```python
from build123d import *

# Parameters (mm, degrees)
SKETCH2_R                     = 30
BOSS_EXTRUDE1_DEPTH           = 20
CUT_EXTRUDE2_DEPTH            = 47.904157598
CUT_EXTRUDE3_START            = -10
CUT_EXTRUDE3_DEPTH            = 10
CBORE_FOR_M3_SHCS1_AT_2_COUNT = 2
CBORE_FOR_M3_SHCS1_AT_2_PITCH = 33.587572106
CBORE_FOR_M3_SHCS1_AT_3_COUNT = 2
CBORE_FOR_M3_SHCS1_AT_3_PITCH = 47.5
SKETCH6_R                     = 2.085
BOSS_EXTRUDE2_DEPTH           = 3


with BuildPart() as part:
    # Sketch2 → Boss-Extrude1 (new body)
    with BuildSketch(Plane(origin=(0, 0, 0), x_dir=(1, 0, 0), z_dir=(0, 1, 0))):
        with Locations(Location((0, 0, 0), (0, 0, 270))):
            Circle(SKETCH2_R)
    extrude(amount=BOSS_EXTRUDE1_DEPTH)

    # Sketch3 → Cut-Extrude2 (cut, through all)
    with BuildSketch(Plane(origin=(0, 20, 0), x_dir=(1, 0, 0), z_dir=(0, 1, 0))):
        with BuildLine():
            ThreePointArc((0, -17.5), (17.5, 0), (0, 17.5))
            Line((0, 17.5), (-2, 17.5))
            Line((-2, 17.5), (-2, 9.2))
            Line((-2, 9.2), (-2, 5.4))
            Line((-2, 5.4), (-8, 0))
            Line((-8, 0), (-2, -5.4))
            Line((-2, -5.4), (-2, -9.2))
            Line((-2, -9.2), (-2, -17.5))
            Line((-2, -17.5), (0, -17.5))
        make_face()
    extrude(amount=-CUT_EXTRUDE2_DEPTH, mode=Mode.SUBTRACT)

    # Sketch3_3 → Cut-Extrude3 (cut)
    with BuildSketch(Plane(origin=(0, 20, 0), x_dir=(1, 0, 0), z_dir=(0, 1, 0)).offset(CUT_EXTRUDE3_START)):
        with BuildLine():
            Line((-17.6, 17.5), (-24.366985862, 17.5))
            ThreePointArc((-24.366985862, 17.5), (-30, 0), (-24.366985862, -17.5))
            Line((-24.366985862, -17.5), (-17.6, -17.5))
            Line((-17.6, -17.5), (-17.6, -21.5))
            Line((-17.6, -21.5), (0, -21.5))
            Line((0, -21.5), (0, -17.5))
            Line((0, -17.5), (-2, -17.5))
            Line((-2, -17.5), (-2, -9.2))
            ThreePointArc((-2, -9.2), (-6.53919762, -12.379149415), (-11.966443699, -13.5))
            Line((-11.966443699, -13.5), (-22, -13.5))
            Line((-22, -13.5), (-22, -9.5))
            Line((-22, -9.5), (-10, -9.5))
            Line((-10, -9.5), (-10, -2))
            Line((-10, -2), (-22, -2))
            Line((-22, -2), (-22, 2))
            Line((-22, 2), (-10, 2))
            Line((-10, 2), (-10, 9.5))
            Line((-10, 9.5), (-22, 9.5))
            Line((-22, 9.5), (-22, 13.5))
            Line((-22, 13.5), (-11.966443699, 13.5))
            ThreePointArc((-11.966443699, 13.5), (-6.53919762, 12.379149415), (-2, 9.2))
            Line((-2, 9.2), (-2, 17.5))
            Line((-2, 17.5), (0, 17.5))
            Line((0, 17.5), (0, 21.5))
            Line((0, 21.5), (-17.6, 21.5))
            Line((-17.6, 21.5), (-17.6, 17.5))
        make_face()
    extrude(amount=CUT_EXTRUDE3_DEPTH, mode=Mode.SUBTRACT)

    # Sketch5 → CBORE for M3 SHCS1 (revolve, cut)
    with BuildSketch(Plane(origin=(0, 0, -23.75), x_dir=(0, 0, -1), z_dir=(1, 0, 0))):
        Polygon((0, 0), (0, 20), (1.7, 20), (1.7, 3), (3.25, 3), (3.25, 0.025), (3.275, 0), align=None)
    cbore_for_m3_shcs1 = revolve(axis=Axis((0, -6.35, -23.75), (0, 1, 0)), mode=Mode.SUBTRACT)

    # CBORE for M3 SHCS1 at 2: CBORE for M3 SHCS1 ×2
    with Locations(*[Vector(0.7071067811865476, 0, 0.7071067811865476) * (i * CBORE_FOR_M3_SHCS1_AT_2_PITCH) for i in range(1, CBORE_FOR_M3_SHCS1_AT_2_COUNT)]):
        add(cbore_for_m3_shcs1, mode=Mode.SUBTRACT)

    # CBORE for M3 SHCS1 at 3: CBORE for M3 SHCS1 ×2
    with Locations(*[(0, 0, i * CBORE_FOR_M3_SHCS1_AT_3_PITCH) for i in range(1, CBORE_FOR_M3_SHCS1_AT_3_COUNT)]):
        add(cbore_for_m3_shcs1, mode=Mode.SUBTRACT)

    # Sketch6 → Boss-Extrude2 (add)
    with BuildSketch(Plane.ZY.offset(10)):
        with Locations((-5.75, 15)):
            Circle(SKETCH6_R)
        with Locations((5.75, 15)):
            Circle(SKETCH6_R)
    extrude(amount=BOSS_EXTRUDE2_DEPTH)


solid = part.part
```
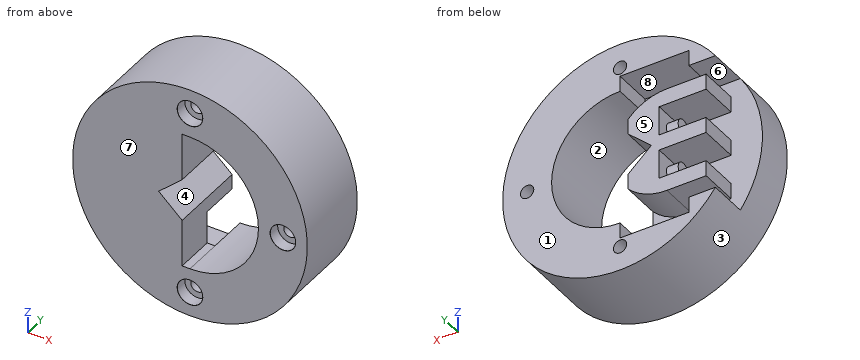
Source: CAD feature listing. Evaluate the final solid. Frame: model axes, mm. Face numbers are marked on the shaded views. A direction names the side the tool comes from. Round coordinates to 2 decimals unless told otherwise and drop trailing zeros. Loops run counter-clockwise (first coordinate to the right, second up) from the corner with the lowest first, then second, coordinate; pieces in that order, holes last.
(1) Section query B-B (y = 7.5). Output: boundary loops of the cut face in (x, z), and give its area (3 significant figures).
From the geometry:
outline: circle Ø60 at (0, 0); hole (-8, 0) - (-2, -5.4) - (-2, -17.5) - (0, -17.5) arc R17.5 ccw to (0, 17.5) - (-2, 17.5) - (-2, 5.4) - close; hole circle Ø3.4 at (0, -23.75); hole circle Ø3.4 at (0, 23.75); hole circle Ø3.4 at (23.75, 0)
area: 2,220 mm2
(2) Section query D-D (x = 23.75). Output: boundary loops of the cut face in (y, z) (3 decimals), and give its area (3 significant figures).
From the geometry:
outline: (0, -18.329) - (20, -18.329) - (20, -1.7) - (3, -1.7) - (3, -3.25) - (0.025, -3.25) - (0, -3.275) - close; (0, 3.275) - (0.025, 3.25) - (3, 3.25) - (3, 1.7) - (20, 1.7) - (20, 18.329) - (0, 18.329) - close
area: 656 mm2
(3) Pull-direction query (X, two-part tool) for the marked faces 1, 2 and 3; classes: +X half, -X half, draft (parallel to the pull), parting line (faces both ways), or undercut.
From the geometry:
face 1: draft
face 2: undercut
face 3: parting line
(4) Contact query for flat-ended pins moving along their axis: pin 1 Ø4 at (x, y) = (-23.5, 8.5) entering from -Z; pin 2 Ø8 at (x, y) = (-17, 15.5) entering from +Z; pin 3 Ø1 at (x, y) = (-15.5, 13.5) entering from -Z. Output: stop coordinate, or through.
From the geometry:
pin 1: stops at z = -20.92
pin 2: stops at z = 27.04
pin 3: stops at z = -25.98
(5) Section query A-A (y = 11.5). Give the number of separate pieces and of enclosed holes in the cut face, and give its area (3 significant figures).
From the geometry:
separate pieces: 2
enclosed holes: 3
area: 1,490 mm2
(6) Access query for the marked faces 4, 5, 6, 7 and 8. Directions: +Z, -Z, +X, -X, +Y, -Y. A direction counts if a zero-diameter tool reaches every point of the face in a straight line with its end or side. Return the directions, or none.
From the geometry:
face 4: +Y, -Y
face 5: +Z, -Z, +X, -X, +Y
face 6: -X, +Y
face 7: +Z, -Z, +X, -X, -Y
face 8: +Y
(7) Section query C-C (z = -15). Output: boundary loops of the cut face in (x, y).
From the geometry:
outline: (-25.98, 0) - (-2, 0) - (-2, 10) - (-25.98, 10) - close; (9.01, 0) - (25.98, 0) - (25.98, 20) - (9.01, 20) - close
(8) Material intervals for probe 1 along Z at (x, y) = (0, 1.55); probe 2 along Z at (x, y) = (0, 9.75); probe 3 along Y at (x, z) = (3, 24), sorted ascending.
From the geometry:
probe 1: z = -30 to -27, -20.5 to -17.5, 17.5 to 20.5, 27 to 30
probe 2: z = -30 to -25.45, -22.05 to -17.5, 17.5 to 22.05, 25.45 to 30
probe 3: y = 3 to 20
